```python
from build123d import *

# Parameters (mm, degrees)
SKETCH1_R           = 6.35
BOSS_EXTRUDE1_DEPTH = 2.54
SKETCH2_R           = 4.8006
BOSS_EXTRUDE2_DEPTH = 7.62
SKETCH3_W           = 4.562763636
SKETCH3_H           = 5.2832
CUT_EXTRUDE1_DEPTH  = 7.62
SKETCH6_R           = 7.62
BOSS_EXTRUDE3_DEPTH = 1.27
SKETCH4_R           = 0.762
CUT_EXTRUDE2_DEPTH  = 4.81
SKETCH5_R           = 0.762
CUT_EXTRUDE3_DEPTH  = 4.81


with BuildPart() as part:
    # Sketch1 → Boss-Extrude1 (new body)
    with BuildSketch(Plane(origin=(0, 0, 0), x_dir=(1, 0, 0), z_dir=(0, 1, 0))):
        Circle(SKETCH1_R)
    extrude(amount=BOSS_EXTRUDE1_DEPTH)

    # Sketch2 → Boss-Extrude2 (add)
    with BuildSketch(Plane(origin=(0, 2.54, 0), x_dir=(1, 0, 0), z_dir=(0, 1, 0))):
        Circle(SKETCH2_R)
    extrude(amount=BOSS_EXTRUDE2_DEPTH)

    # Sketch3 → Cut-Extrude1 (cut)
    with BuildSketch(Plane(origin=(0, 10.16, 0), x_dir=(1, 0, 0), z_dir=(0, 1, 0))):
        Rectangle(SKETCH3_W, SKETCH3_H)
    extrude(amount=-CUT_EXTRUDE1_DEPTH, mode=Mode.SUBTRACT)

    # Sketch6 → Boss-Extrude3 (add)
    with BuildSketch(Plane.XZ):
        Circle(SKETCH6_R)
    extrude(amount=BOSS_EXTRUDE3_DEPTH)

    # Sketch4 → Cut-Extrude2 (cut, through all)
    with BuildSketch(Plane(origin=(0, 2.54, 0), x_dir=(1, 0, 0), z_dir=(0, 1, 0))):
        with Locations((0, -1.27)):
            Circle(SKETCH4_R)
    extrude(amount=-CUT_EXTRUDE2_DEPTH, mode=Mode.SUBTRACT)

    # Sketch5 → Cut-Extrude3 (cut, through all)
    with BuildSketch(Plane(origin=(0, 2.54, 0), x_dir=(1, 0, 0), z_dir=(0, 1, 0))):
        with Locations((0, 1.27)):
            Circle(SKETCH5_R)
    extrude(amount=-CUT_EXTRUDE3_DEPTH, mode=Mode.SUBTRACT)


solid = part.part
```
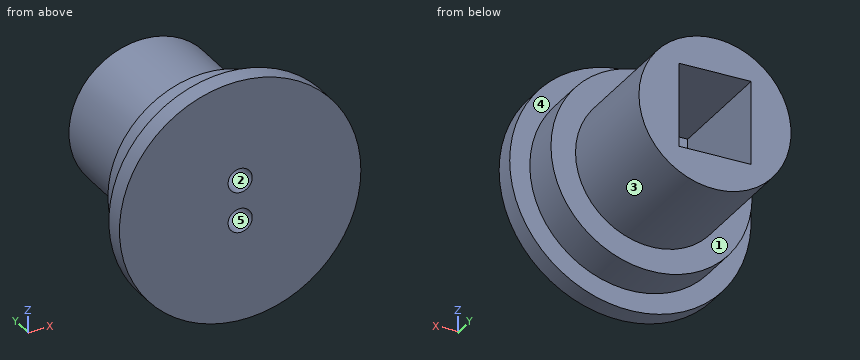
Read the model definition and answer for the solid it produces. Units are mm, in the model's axes. Face numbers are marked on the shaded views. A direction names the side the tool comes from. Round coordinates to 2 decimals unless told otherwise and drop trailing zeros. Write each loop counter-clockwise with the first axis right and the second up, starting at its lowest first coordinate (ties: lowest second). Pieces come first, ordered by that corner, then holes. Notation, with made-up numbers: (-10.75, 75) - (17.25, 75) arc R7 ccw to (17.25, 87) - close; hole circle Ø2 at (71, 10). An arc over 180 degrees is marked (long way). One line per item, written item: value.
Q1. Which of the six approach directions +Z, -Z, +X, -X, +Y, -Y give full straight-line access (tool end or side, diameter ignored) to the marked faces 4 and 5?
The answers:
face 4: +Y
face 5: +Y, -Y
Q2. Find section C-C (y = 6). Determine the outline of the cut face in (x, z).
The answers:
outline: circle Ø9.6 at (0, 0); hole (-2.28, -2.64) - (2.28, -2.64) - (2.28, 2.64) - (-2.28, 2.64) - close
Q3. For a pull along Z with two mould halves and no side action, classify the marked faces 1, 2 and 3 as pulls with the +Z half, pulls with the -Z half, needs draft (parallel to the pull), parting line crosses it, or undercut.
The answers:
face 1: needs draft
face 2: undercut
face 3: parting line crosses it
Q4. Find section D-D (z = -3.5). Determine the outline of the cut face in (x, y).
The answers:
outline: (-6.77, -1.27) - (6.77, -1.27) - (6.77, 0) - (5.3, 0) - (5.3, 2.54) - (3.29, 2.54) - (3.29, 10.16) - (-3.29, 10.16) - (-3.29, 2.54) - (-5.3, 2.54) - (-5.3, 0) - (-6.77, 0) - close
Q5. Find section B-B (z = -1.27). Determine the outline of the cut face in (x, y), and give its area (3 significant figures).
The answers:
outline: (-7.51, -1.27) - (-0.76, -1.27) - (-0.76, 2.54) - (-2.28, 2.54) - (-2.28, 10.16) - (-4.63, 10.16) - (-4.63, 2.54) - (-6.22, 2.54) - (-6.22, 0) - (-7.51, 0) - close; (0.76, -1.27) - (7.51, -1.27) - (7.51, 0) - (6.22, 0) - (6.22, 2.54) - (4.63, 2.54) - (4.63, 10.16) - (2.28, 10.16) - (2.28, 2.54) - (0.76, 2.54) - close
area: 80.7 mm2
Q6. Each of these flat-tipped pins is pushed along its axis until it touches: P1, Ø1, axis at y = 3.5, z = 3, coming from the +X side; P2, Ø1, axis at x = -5.5, z = -5, coming from the +Y side; P3, Ø3.5, axis at x = -0.5, y = 8, coming from the -Z side; P4, Ø1.2, axis at x = 0, z = -1.27, coming from the -Y side. Where does it stop, or does it pass through?
The answers:
P1: stops at x = 4.1
P2: stops at y = 0
P3: stops at z = -4.8
P4: passes through
Q7. Straight lines are drawn through the part: line 1 (Z direction, x = 0, y = -0.1); line 2 (Z direction, x = 0, y = 0.1); line 3 (X direction, y = 1.25, z = -1.27). For each, find the intervals that lie inside material, in ascending order. Write a range as from..to.
The answers:
line 1: z = -7.62..-2.03, -0.51..0.51, 2.03..7.62
line 2: z = -6.35..-2.03, -0.51..0.51, 2.03..6.35
line 3: x = -6.22..-0.76, 0.76..6.22
Q8. Find section A-A (x = 0). Determine the outline of the cut face in (y, z).
The answers:
outline: (-1.27, -7.62) - (0, -7.62) - (0, -6.35) - (2.54, -6.35) - (2.54, -4.8) - (10.16, -4.8) - (10.16, -2.64) - (2.54, -2.64) - (2.54, -2.03) - (-1.27, -2.03) - close; (-1.27, -0.51) - (2.54, -0.51) - (2.54, 0.51) - (-1.27, 0.51) - close; (-1.27, 2.03) - (2.54, 2.03) - (2.54, 2.64) - (10.16, 2.64) - (10.16, 4.8) - (2.54, 4.8) - (2.54, 6.35) - (0, 6.35) - (0, 7.62) - (-1.27, 7.62) - close
